from build123d import *

# Parameters (mm, degrees)
F0_W     = 70
F0_H     = 40
F1_DEPTH = 30
F3_DEPTH = 20
F4_W     = 25
F4_H     = 30
F5_DEPTH = 30.001


with BuildPart() as f1:
    # F0 (on Front) → F1 (new body)
    with BuildSketch(Plane.XZ):
        Rectangle(F0_W, F0_H)
    extrude(amount=F1_DEPTH)

    # F2 (on face) → F3 (cut)
    with BuildSketch(Plane.XZ.offset(30)):
        Polygon((35, 0), (35, 20), (0, 20), (0, 4.09944), (0, 0), (0, -10), (35, -10), align=None)
    extrude(amount=-F3_DEPTH, mode=Mode.SUBTRACT)

    # F4 (on face) → F5 (cut, through all)
    with BuildSketch(Plane.XZ.offset(30)):
        with Locations((-22.5, -5)):
            Rectangle(F4_W, F4_H)
    extrude(amount=-F5_DEPTH, mode=Mode.SUBTRACT)


solid = f1.part
Model file for the job. Use its own axes, mm. A direction names the side the tool comes from. Give positions to 0.01 mm unless a question says otherwise; leave off trailing zeros. Loops run counter-clockwise (first coordinate to the right, second up) from the corner with the lowest first, then second, coordinate; pieces in that order, holes last.
Item 1: Slice it at C-C (x = 21). Write the cut outline in (y, z), plus the area to 3 significant figures.
Check values:
outline: (-30, -20) - (0, -20) - (0, 20) - (-10, 20) - (-10, -10) - (-30, -10) - close
area: 600 mm2
Item 2: Slice it at A-A (y = -21.25). Write the cut outline in (x, z).
Check values:
outline: (-35, 10) - (-10, 10) - (-10, -20) - (35, -20) - (35, -10) - (0, -10) - (0, 20) - (-35, 20) - close
Item 3: Slice it at B-B (z = 13). Write the cut outline in (x, y), plus the area to 3 significant figures.
Check values:
outline: (-35, -30) - (0, -30) - (0, -10) - (35, -10) - (35, 0) - (-35, 0) - close
area: 1,400 mm2
Item 4: Drop flat-ended pins along their axis: P1, Ø10, axis at y = -21, z = 4.5, coming from the +X side; P2, Ø2, axis at y = -12, z = 3, coming from the -X side. Give the stop position or say it passes through.
Check values:
P1: stops at x = 0
P2: stops at x = -10
Item 5: Slice it at D-D (z = -12.5). Write the cut outline in (x, y).
Check values:
outline: (-10, -30) - (35, -30) - (35, 0) - (-10, 0) - close
Item 6: Which spindle directions (+Z, -Z, +X, -X, +Y, -Y) get a long thin tool onto all of the face, cutting with end or side? Do faces 1 (the face through (-35, -15, 15)), 2 (the face through (-23, -15, 10)), 3 (the face through (17, -20, -10)). Say none if no direction does.
Check values:
face 1: +Z, -Z, -X, +Y, -Y
face 2: -Z, -X, +Y, -Y
face 3: +Z, +X, -Y
Item 7: Drill centre lines: line 1 along X through (y, z) = (-18.75, 1); line 2 along X through (y, z) = (-20.25, -14); line 3 along Z through (x, y) = (18, -25.25). Where is each one in solid material? Low to high.
Check values:
line 1: x = -10 to 0
line 2: x = -10 to 35
line 3: z = -20 to -10
